Geometry: final body of the model. Coordinates: model frame, mm. A direction names the side the tool comes from. Give positions to 0.01 mm unless a question says otherwise; leave off trailing zeros. Write each loop counter-clockwise with the first axis right and the second up, starting at its lowest first coordinate (ties: lowest second). Pieces come first, ordered by that corner, then holes. Notation, with made-up numbers: (67, 58.25) - (117, 58.25) arc R4 cw to (117, 62.25) - close; hole circle Ø8 at (82.5, 85). An arc over 180 degrees is marked (long way). Return JSON: item names as keys, results as strings.
from build123d import *

# Parameters (mm, degrees)
LOFT1_OUTLINE_W     = 204.216
LOFT1_OUTLINE_H     = 204.216
LOFT1_DEPTH         = 1021.439287055
LOFT1_DRAFT         = -1.324797
SKETCH3_2_W         = 251.46
SKETCH3_2_H         = 251.46
BOSS_EXTRUDE1_DEPTH = 306.324
SKETCH2_2_W         = 204.216
SKETCH2_2_H         = 204.216
BOSS_EXTRUDE2_DEPTH = 306.324


# Read off the part's stored shape, not the designer's step: Loft1
with BuildPart() as part:
    # Loft1 outline → Loft1 (with draft: the straight prism first)
    with BuildSketch(Plane.YZ.offset(-0.580963743)):
        Rectangle(LOFT1_OUTLINE_W, LOFT1_OUTLINE_H)
    extrude(amount=LOFT1_DEPTH)
    # Loft1: the draft: its side faces are tilted about the plane it starts from
    loft1_sides = [part.faces().sort_by_distance(p)[0] for p in [
        (510.138679785, 102.108, 0),
        (510.138679785, 0, 102.108),
        (510.138679785, -102.108, 0),
        (510.138679785, 0, -102.108),
    ]]
    draft(loft1_sides, Plane.YZ.offset(-0.580963743), LOFT1_DRAFT)

    # Sketch3<2> → Boss-Extrude1 (add)
    with BuildSketch(Plane(origin=(1020.858323313, 0, 0), x_dir=(0, 0, -1), z_dir=(1, 0, 0))):
        Rectangle(SKETCH3_2_W, SKETCH3_2_H)
    extrude(amount=BOSS_EXTRUDE1_DEPTH)

    # Sketch2<2> → Boss-Extrude2 (add)
    with BuildSketch(Plane(origin=(-0.580963743, 0, 0), x_dir=(0, 0, -1), z_dir=(1, 0, 0))):
        Rectangle(SKETCH2_2_W, SKETCH2_2_H)
    extrude(amount=-BOSS_EXTRUDE2_DEPTH)


solid = part.part
Q1. Section query D-D, the plane x = 412.5. Return the cut outline in (y, z).
Answer key:
{"outline": "(-111.66, -111.66) - (111.66, -111.66) - (111.66, 111.66) - (-111.66, 111.66) - close"}
Q2. Section query A-A, the plane z = -40.5. Return the cut outline in (x, y), plus the area to 3 significant figures.
Answer key:
{"outline": "(-306.9, -102.11) - (-0.58, -102.11) - (1020.86, -125.73) - (1327.18, -125.73) - (1327.18, 125.73) - (1020.86, 125.73) - (-0.58, 102.11) - (-306.9, 102.11) - close", "area": "372,000 mm^2"}
Q3. Material intervals for probe 1 along Y at (x, z) = (-17, 7); probe 2 along Y at (x, z) = (804, -34), sorted ascending. Write a range as [from, to].
Answer key:
{"probe 1": "y = [-102.11, 102.11]", "probe 2": "y = [-120.71, 120.71]"}
Q4. Section query C-C, the plane x = -93.5. Return the cut outline in (y, z).
Answer key:
{"outline": "(-102.11, -102.11) - (102.11, -102.11) - (102.11, 102.11) - (-102.11, 102.11) - close"}
Q5. Set-up query: faces 1 (the flat face through (-152, -1, -102.108)), 2 (the flat face through (-152, -1, 102.108)), 3 (the flat face through (-152, 102.108, 1)), 4 (the flat face through (-152, -102.108, 1)), 5 (the flat face through (1172, -125.73, 2)). Return all of +Z, -Z, +X, -X, +Y, -Y with unobstructed straight access to the full face (end or side cutting, diameter ignored); none if empty.
Answer key:
{"face 1": "-Z, -X, +Y, -Y", "face 2": "+Z, -X, +Y, -Y", "face 3": "+Z, -Z, -X, +Y", "face 4": "+Z, -Z, -X, -Y", "face 5": "+Z, -Z, +X, -X, -Y"}
Q6. Pin query (flat end, axial travel): P1, Ø12, axis at x = 49.5, y = -49, coming from the -Z side; P2, Ø2, axis at x = 355.5, z = -67.5, coming from the -Y side; P3, Ø5, axis at x = -90.5, y = 21, coming from the +Z side. Return the tip coordinate at first contact, or that it passes through.
Answer key:
{"P1": "stops at z = -103.4", "P2": "stops at y = -110.37", "P3": "stops at z = 102.11"}
